Can you work these out from the model? Positions are in its coordinate system, mm. A direction names the side the tool comes from. Coordinates: 2 decimals unless noted, no trailing zeros. Order: outer loops, then holes, each group sorted by start corner. A loop starts at its lowest first (then second) coordinate and runs counter-clockwise, first axis right, second up. Notation, with made-up numbers: (-33, 7.5) -> (-16, 7.5) arc R18 ccw to (-16, 40.5) -> close; hole circle Ø1 at (-30, 4). An arc over 180 degrees is marked (long way). Answer in a Markdown table with one row per item. Add a question column.
1. On a 3-axis mill with a long thin cutter (end or side, diameter ignored), from which of +Z, -Z, +X, -X, +Y, -Y can I reach the whole of each face in a straight line? I mean faces 4 (the face through (-4.028, -0.047, 21.423)), 5 (the face through (0, 0, 0)). Say none if no direction works.
2. If I drill on line 1 along Z through (x, y) = (-4.4, 0); line 2 along Y through (x, z) = (0, 23.75), over which ranges is the centre line in solid material (lowest first)? Write a range as [from, to].
3. We'd pull the mould along X, two halves only. Please class faces 1 (the face through (-3, 1, 30)), 2 (the face through (2.44, 0.54, 24.68)), 3 (the face through (6.057, -1.907, 14.797)): pulls with the +X half, pulls with the -X half, needs draft (parallel to the pull), parting line crosses it, or undercut.
4. Imagine slicing it at A-A on z = 25.5. Write out the boundary of the cut face in (x, y), plus the area to 3 significant figures.
5. Will these pins go through, and if not, where does the flat tip stop? pin 1 (2 mm diameter, centred on y = -3, z = 8.5, fed in from -X); pin 2 (4.5 mm diameter, centred on x = 0, y = 0, fed in from +Z); pin 3 (1.3 mm diameter, centred on y = 0, z = 27.5, fed in from -X).
6. Imagine slicing it at B-B on z = 18. Write out the boundary of the cut face in (x, y), plus the area to 3 significant figures.
7. Imagine slicing it at C-C on x = -4.75. State how many separate pieces and enclosed holes the cut face has, plus the area to 3 significant figures.
Autodesk Inventor part; units mm, degrees
ref_plane "Work Plane1" through (-6.35, 0, 0) normal (1, 0, 0) x (0, 1, 0)
ref_plane "XZ Plane" through (0, 0, 0) normal (0, 1, 0) x (-1, 0, 0)
ref_plane "XY Plane" through (0, 0, 0) normal (0, 0, 1) x (1, 0, 0)
sketch "Sketch1" plane through (0, 0, 0) normal (0, 0, 1) x (1, 0, 0)
  circle A0 centre (0, 0) radius 6.35
  dimension "d0" = 12.7
extrude "Extrusion1" add sketch "Sketch1" along normal blind 30
hole "Hole1" at (0, 0, 30) direction (0, 0, -1) diameter 5 depth 10 tip angle 118
fillet "Fillet1" radius 0.5 3 edges at (0, 2.5, 30) (-6.35, 0, 30) (-6.35, 0, 0)
ref_plane "Work Plane1" through (-6.35, 0, 0) normal (1, 0, 0) x (0, 1, 0)
sketch "Sketch2" plane through (-6.35, 0, 0) normal (1, 0, 0) x (0, 1, 0)
  line L0 (0, 50.0021) -> (0, 0) construction
  line L1 (-5.85, 30) -> (5.85, 30) construction
  point P0 (0, 27.5)
  point P1 (0, 22.5)
  dimension "d23" = 2.5
  dimension "d24" = 5
hole "Hole3" at (-6.35, 0, 27.5) at (-6.35, 0, 22.5) direction (1, 0, 0) diameter 2.156 end up to surface
fillet "Fillet2" radius 0.5 4 edges at (-6.2578, 1.078, 27.4975) (-6.2578, -1.078, 27.4972) (-6.2578, 1.078, 22.4975) (-6.2578, -1.078, 22.4972)
properties part number "Roller" material "Nylon-6/6"
Answers follow:
| question | item | result |
|---|---|---|
| 1 | face 4 | -X |
| 1 | face 5 | -Z, +X, -X, +Y, -Y |
| 2 | line 1 | z = [0, 21.42], [23.58, 26.42], [28.58, 30] |
| 2 | line 2 | y = [-6.35, -2.5], [2.5, 6.35] |
| 3 | face 1 | needs draft |
| 3 | face 2 | undercut |
| 3 | face 3 | parting line crosses it |
| 4 | outline | circle Ø12.7 at (0, 0); hole circle Ø5 at (0, 0) |
| 4 | area | 107 mm² |
| 5 | pin 1 | stops at x = -6.03 |
| 5 | pin 2 | stops at z = 19.85 |
| 5 | pin 3 | stops at x = 2.41 |
| 6 | outline | circle Ø12.7 at (0, 0) |
| 6 | area | 127 mm² |
| 7 | separate pieces | 1 |
| 7 | enclosed holes | 2 |
| 7 | area | 245 mm² |
